Source: CAD feature listing. Evaluate the final solid. Frame: model axes, mm. Face numbers are marked on the shaded views. Give positions to 0.01 mm unless a question says otherwise; leave off trailing zeros. Loops run counter-clockwise (first coordinate to the right, second up) from the corner with the lowest first, then second, coordinate; pieces in that order, holes last. Notation, with made-up numbers: (59.25, -33.75) - (94.25, -33.75) arc R6 cw to (94.25, -29.75) - close; hole circle Ø5 at (-16, 21). An arc over 180 degrees is marked (long way). Put each result on its own line as item: value.
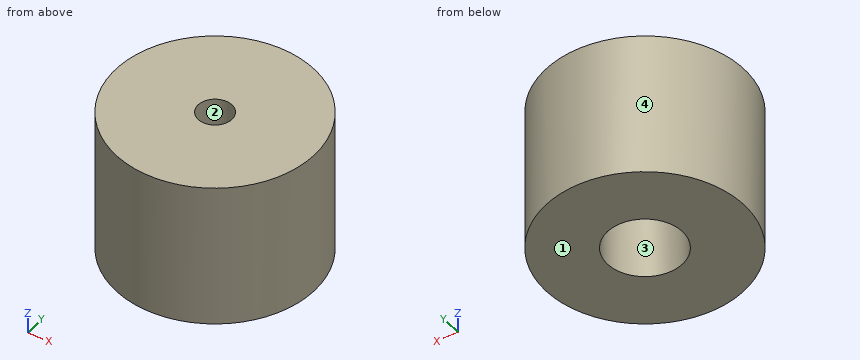
Autodesk Inventor part; units mm, degrees
ref_plane "YZ Plane" through (0, 0, 0) normal (1, 0, 0) x (0, 1, 0)
ref_plane "XZ Plane" through (0, 0, 0) normal (0, 1, 0) x (-1, 0, 0)
ref_plane "XY Plane" through (0, 0, 0) normal (0, 0, 1) x (1, 0, 0)
sketch "Skizze1" plane through (0, 0, 0) normal (0, 0, 1) x (1, 0, 0)
  circle A0 centre (0, 0) radius 18.5
  dimension "d0" = 37
extrude "Extrusion1" add sketch "Skizze1" along normal blind 27
sketch "Skizze2" plane through (0, 0, 0) normal (0, 0, -1) x (-1, 0, 0)
  circle A0 centre (0, 0) radius 7
  dimension "d3" = 14
extrude "Extrusion2" cut sketch "Skizze2" against normal blind 12
sketch "Skizze3" plane through (0, 0, 12) normal (0, 0, -1) x (-1, 0, 0)
  point P0 (0, 0)
hole "Bohrung1" at (0, 0, 12) direction (0, 0, 1) diameter 6.3 end through all
properties part number "GummiFeet" material "Gummi, Silikon"
1) Mould query, pull axis Y, two halves, no side actions, for the marked faces 1, 2, 3 and 4. Classes: pulls with the +Y half, pulls with the -Y half, needs draft (parallel to the pull), parting line crosses it, or undercut.
Check result:
face 1: needs draft
face 2: undercut
face 3: undercut
face 4: parting line crosses it
2) Section query C-C, the plane x = 6.5. Output: boundary loops of the cut face in (y, z), plus the area to 3 significant figures.
Check result:
outline: (-17.32, 0) - (-2.6, 0) - (-2.6, 12) - (2.6, 12) - (2.6, 0) - (17.32, 0) - (17.32, 27) - (-17.32, 27) - close
area: 873 mm²
3) Pin query (flat end, axial travel): P1, Ø5, axis at y = 4.5, z = 7, coming from the +X side; P2, Ø12, axis at y = 13, z = 13, coming from the +X side; P3, Ø8, axis at x = 6, z = 11.5, coming from the -Y side; P4, Ø5.5, axis at x = 0, y = 0, coming from the +Z side. Return the tip coordinate at first contact, or that it passes through.
Check result:
P1: x = 18.39
P2: x = 17.12
P3: y = -18.39
P4: through
4) Material intervals for line 1 along Y through (x, z) = (0, 6.5); line 2 along Y through (x, z) = (0, 21); line 3 along X through (y, z) = (2, 13), sorted ascending. Write a range as [from, to].
Check result:
line 1: [-18.5, -7], [7, 18.5]
line 2: [-18.5, -3.15], [3.15, 18.5]
line 3: [-18.39, -2.43], [2.43, 18.39]
5) Section query D-D, the plane z = 6. Output: boundary loops of the cut face in (x, y), plus the area to 3 significant figures.
Check result:
outline: circle Ø37 at (0, 0); hole circle Ø14 at (0, 0)
area: 921 mm²
6) Section query A-A, the plane x = 0. Output: boundary loops of the cut face in (y, z), plus the area to 4 significant figures.
Check result:
outline: (-18.5, 0) - (-7, 0) - (-7, 12) - (-3.15, 12) - (-3.15, 27) - (-18.5, 27) - close; (3.15, 12) - (7, 12) - (7, 0) - (18.5, 0) - (18.5, 27) - (3.15, 27) - close
area: 736.5 mm²
